The listing builds one solid part. Answer for the finished solid, in the listing's coordinates (mm). Face numbers are marked on the shaded views. Round coordinates to 2 decimals unless told otherwise and drop trailing zeros. Loops run counter-clockwise (first coordinate to the right, second up) from the corner with the lowest first, then second, coordinate; pieces in that order, holes last. Notation, with made-up numbers: (21, 77) -> (38, 77) arc R30 ccw to (38, 107) -> close; hole circle Ø9 at (19.5, 85). An arc over 180 degrees is marked (long way). Use a Markdown table: item, result. Add a question column.
Q1. For a pull along Y with two mould halves and no side action, classify the marked faces 1 and 2 as released by +Y, released by -Y, zero draft, split by the parting line, or undercut.
Q2. Section C-C on z = -9 is taken. Give the vertices of the cut face in (x, y), then the cut area to 3 significant figures.
Q3. Section A-A on x = 0 is taken. Give the vertices of the cut face in (y, z), then the cut area to 3 significant figures.
Q4. Consider line 1 (Y direction, x = 0, z = 5); line 2 (X direction, y = -0.5, z = 1); line 3 (Y direction, x = -0.75, z = -2). Determine where each line is inside the solid, lowest interval first.
Q5. Given pin 1 Ø1 at (x, z) = (-2.5, 6) entering from +Y; pin 2 Ø2 at (x, z) = (3, -15.5) entering from -Y, each flat-ended and moving along its own axis, determine where each tip first touches the part or whether it passes through.
from build123d import *

# Parameters (mm, degrees)
SKETCH1_R               = 3.8
BOSS_EXTRUDE1_DEPTH     = 20
SKETCH2_R               = 2
CUT_EXTRUDE1_DEPTH      = 21
CUT_EXTRUDE1_DEPTH_BACK = 21
FILLET1_R               = 0.8


with BuildPart() as part:
    # Sketch1 → Boss-Extrude1 (new body, symmetric)
    with BuildSketch(Plane.XY):
        Circle(SKETCH1_R)
    extrude(amount=BOSS_EXTRUDE1_DEPTH, both=True)

    # Sketch2 → Cut-Extrude1 (cut, two sides)
    with BuildSketch(Plane.XY) as cut_extrude1_sk:
        Circle(SKETCH2_R)
    extrude(amount=CUT_EXTRUDE1_DEPTH, mode=Mode.SUBTRACT)
    extrude(cut_extrude1_sk.sketch, amount=-CUT_EXTRUDE1_DEPTH_BACK, mode=Mode.SUBTRACT)

    # Fillet1
    fillet1_edges = [part.edges().sort_by_distance(p)[0] for p in [
        (-3.8, 0, 20),
    ]]
    fillet(fillet1_edges, radius=FILLET1_R)


solid = part.part
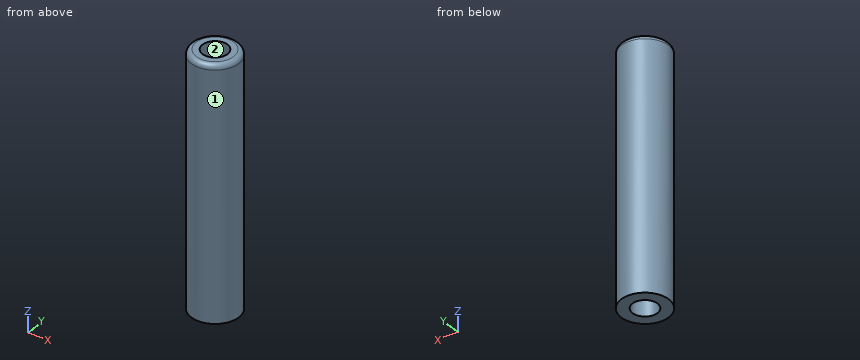
Checked values:
| question | item | result |
|---|---|---|
| 1 | face 1 | split by the parting line |
| 1 | face 2 | undercut |
| 2 | outline | circle Ø7.6 at (0, 0); hole circle Ø4 at (0, 0) |
| 2 | area | 32.8 mm2 |
| 3 | outline | (-3.8, -20) -> (-2, -20) -> (-2, 20) -> (-3, 20) arc R0.8 ccw to (-3.8, 19.2) -> close; (2, -20) -> (3.8, -20) -> (3.8, 19.2) arc R0.8 ccw to (3, 20) -> (2, 20) -> close |
| 3 | area | 144 mm2 |
| 4 | line 1 | y = -3.8 to -2, 2 to 3.8 |
| 4 | line 2 | x = -3.77 to -1.94, 1.94 to 3.77 |
| 4 | line 3 | y = -3.73 to -1.85, 1.85 to 3.73 |
| 5 | pin 1 | stops at y = 3.23 |
| 5 | pin 2 | stops at y = -3.23 |
